Input: part model. Units: mm. Frame: model coordinates. Coordinates: 2 decimals unless noted, no trailing zeros. Loops run counter-clockwise (first coordinate to the right, second up) from the corner with the lowest first, then second, coordinate; pieces in that order, holes last.
(1) Section A-A, the plane y = 0. Return loops of the section in (x, z).
(2) Section B-B, the plane x = 0. Return loops of the section in (y, z), then the cut area to 4 significant figures.
(3) Contact query for a flat-ended pin moving along its axis: P1, Ø10, axis at x = 0, y = 0, coming from the +Z side. Output: stop coordinate, or through.
(4) Section D-D, the plane z = 1.4. Return loops of the section in (x, y), then the cut area to 3 significant figures.
(5) Line query: L1, parallel to Y at x = 37.5, z = 3; L2, parallel to Y at x = 0, z = 1.5; L3, parallel to X at y = 2, z = 4.2. Output: solid intervals per line, ascending.
(6) Section C-C, the plane y = 20.5. Return loops of the section in (x, z), then the cut area to 3 significant figures.
(7) Mould query, pull axis Y, two halves, no side actions, for faces 1 (the face through (45, 0, 2)), 2 (the face through (-36.6, -19, 2.5)), 3 (the face through (-1, -28, 2)). Classes: released by +Y, released by -Y, zero draft, split by the parting line, or undercut.
```python
from build123d import *

# Parameters (mm, degrees)
SKETCH_1_W          = 90
SKETCH_1_H          = 56
SKETCH_1_R          = 1.75
EXTRUDE_1_DEPTH     = 5
SKETCH_2_R          = 8.25
CUT_EXTRUDE_1_DEPTH = 5


with BuildPart() as part:
    # ｽｹｯﾁ1 → ﾎﾞｽ - 押し出し1 (new body)
    with BuildSketch(Plane.XY):
        Rectangle(SKETCH_1_W, SKETCH_1_H)
        with Locations((-37.5, 20.5)):
            Circle(SKETCH_1_R, mode=Mode.SUBTRACT)
        with Locations((37.5, 20.5)):
            Circle(SKETCH_1_R, mode=Mode.SUBTRACT)
        with Locations((37.5, -20.5)):
            Circle(SKETCH_1_R, mode=Mode.SUBTRACT)
        with Locations((-37.5, -20.5)):
            Circle(SKETCH_1_R, mode=Mode.SUBTRACT)
    extrude(amount=EXTRUDE_1_DEPTH)

    # ｽｹｯﾁ2 → ｶｯﾄ - 押し出し1 (cut)
    with BuildSketch(Plane.XY.offset(5)):
        Circle(SKETCH_2_R)
    extrude(amount=-CUT_EXTRUDE_1_DEPTH, mode=Mode.SUBTRACT)


solid = part.part
```
Report:
1. outline: (-45, 0) - (-8.25, 0) - (-8.25, 5) - (-45, 5) - close; (8.25, 0) - (45, 0) - (45, 5) - (8.25, 5) - close
2. outline: (-28, 0) - (-8.25, 0) - (-8.25, 5) - (-28, 5) - close; (8.25, 0) - (28, 0) - (28, 5) - (8.25, 5) - close
2. area: 197.5 mm2
3. P1: passes through
4. outline: (-45, -28) - (45, -28) - (45, 28) - (-45, 28) - close; hole circle Ø3.5 at (-37.5, -20.5); hole circle Ø3.5 at (-37.5, 20.5); hole circle Ø16.5 at (0, 0); hole circle Ø3.5 at (37.5, -20.5); hole circle Ø3.5 at (37.5, 20.5)
4. area: 4,790 mm2
5. L1: y = -28 to -22.25, -18.75 to 18.75, 22.25 to 28
5. L2: y = -28 to -8.25, 8.25 to 28
5. L3: x = -45 to -8, 8 to 45
6. outline: (-45, 0) - (-39.25, 0) - (-39.25, 5) - (-45, 5) - close; (-35.75, 0) - (35.75, 0) - (35.75, 5) - (-35.75, 5) - close; (39.25, 0) - (45, 0) - (45, 5) - (39.25, 5) - close
6. area: 415 mm2
7. face 1: zero draft
7. face 2: undercut
7. face 3: released by -Y
